Could you check a few things on this model? Use its own coordinates, in mm. A direction names the side the tool comes from. Round coordinates to 2 decimals unless told otherwise and drop trailing zeros. Loops run counter-clockwise (first coordinate to the right, second up) from the corner with the lowest first, then second, coordinate; pieces in that order, holes last. Notation, with made-up numbers: M 12.5,-8.75 L 46.5,-8.75 A30 cw 46.5,15.25 Z; hole C 72.25,23 d8. An arc over 180 degrees is marked long. Answer in a Markdown table with one row per item.
```python
from build123d import *

# Parameters (mm, degrees)
SKETCH1_R           = 11
SKETCH1_R_2         = 4
BOSS_EXTRUDE1_DEPTH = 7
SKETCH2_R           = 9.8
SKETCH2_R_2         = 6
CUT_EXTRUDE1_DEPTH  = 0.2
FILLET1_R           = 0.2


with BuildPart() as part:
    # Sketch1 → Boss-Extrude1 (new body)
    with BuildSketch(Plane.XY):
        Circle(SKETCH1_R)
        Circle(SKETCH1_R_2, mode=Mode.SUBTRACT)
    extrude(amount=BOSS_EXTRUDE1_DEPTH)

    # Sketch2 → Cut-Extrude1 (cut)
    with BuildSketch(Plane.XY.offset(7)):
        Circle(SKETCH2_R)
        Circle(SKETCH2_R_2, mode=Mode.SUBTRACT)
    cut_extrude1 = extrude(amount=-CUT_EXTRUDE1_DEPTH, mode=Mode.SUBTRACT)

    # Mirror1: Cut-Extrude1 across plane
    add(cut_extrude1.mirror(Plane.XY.offset(3.5)), mode=Mode.SUBTRACT)

    # Fillet1
    fillet1_edges = [part.edges().sort_by_distance(p)[0] for p in [
        (-11, 0, 0),
        (-11, 0, 7),
        (-4, 0, 0),
        (-4, 0, 7),
    ]]
    fillet(fillet1_edges, radius=FILLET1_R)


solid = part.part
```
1) If we mould it in two halves opening along Y, with no side actions, what happens to faces 4 (the face through (-2.38, -10.74, 3.45)), 5 (the face through (-0.867, -3.905, 3.454)), 6 (the face through (3, -4, 0))? For each: released by +Y, released by -Y, zero draft, split by the parting line, or undercut.
Computed:
| item | result |
|---|---|
| face 4 | split by the parting line |
| face 5 | undercut |
| face 6 | zero draft |
2) Which directions (+Z, -Z, +X, -X, +Y, -Y) give clear straight access to the entire face, cutting with the end or side of a thin tool? Please do faces 1 (the face through (3, -4, 7)), 2 (the face through (4.2, 4.5, 6.8)), 3 (the face through (4.2, 4.5, 0.2)).
Computed:
| item | result |
|---|---|
| face 1 | +Z, +X, -X, +Y, -Y |
| face 2 | +Z |
| face 3 | -Z |
3) I need wall thicknesses on line 1 (Y direction, x = 0, z = 0.15); line 2 (Z direction, x = 6.5, y = 4.75); line 3 (Y direction, x = -3, z = 6.5). Which ranges of each line are inside material? Lowest first, please.
Computed:
| item | result |
|---|---|
| line 1 | y = -10.99 to -9.8, -6 to -4.01, 4.01 to 6, 9.8 to 10.99 |
| line 2 | z = 0.2 to 6.8 |
| line 3 | y = -10.58 to -2.65, 2.65 to 10.58 |
4) I want a section at C-C, the plane z = 2. Please give me the cut outline in (x, y).
Computed:
| item | result |
|---|---|
| outline | C 0,0 d22; hole C 0,0 d8 |
5) Will these pins go through, and if not, where does the flat tip stop? P1, Ø3, axis at x = 8.5, z = 4, coming from the -Y side; P2, Ø7, axis at x = 0, y = 0, coming from the -Z side; P3, Ø2, axis at x = 5, z = 3.5, coming from the +Y side; P4, Ø1.5, axis at y = -5.5, z = 6, coming from the +X side.
Computed:
| item | result |
|---|---|
| P1 | stops at y = -8.49 |
| P2 | passes through |
| P3 | stops at y = 10.25 |
| P4 | stops at x = 9.92 |
